Autodesk Inventor part; units mm, degrees
ref_plane "YZ Plane" through (0, 0, 0) normal (1, 0, 0) x (0, 1, 0)
ref_plane "XZ Plane" through (0, 0, 0) normal (0, 1, 0) x (-1, 0, 0)
ref_plane "XY Plane" through (0, 0, 0) normal (0, 0, 1) x (1, 0, 0)
sketch "Esboço1" plane through (0, 0, 0) normal (0, 1, 0) x (-1, 0, 0)
  line L0 (2.5876, 3.6816) -> (2.5876, -3.6816)
  line L1 (-2.5876, 3.6816) -> (-2.5876, -3.6816)
  arc A0 (2.5876, 3.6816) -> (-2.5876, 3.6816) centre (0, 0) ccw
  arc A1 (-2.5876, -3.6816) -> (2.5876, -3.6816) centre (0, 0) ccw
extrude "Extrusão1" add sketch "Esboço1" along normal blind 0.3
sketch "Esboço2" plane through (0, 0.3, 0) normal (0, 1, 0) x (1, 0, 0)
  circle A0 centre (0, 0) radius 3.5
  dimension "d3" = 7
extrude "Extrusão2" add sketch "Esboço2" along normal blind 5
properties part number "button"
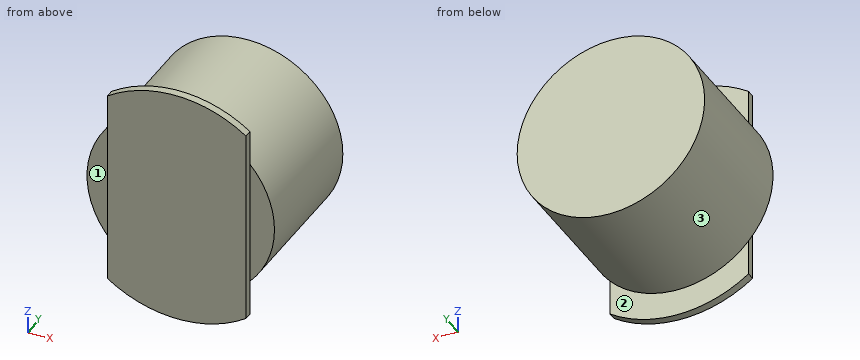
Design review of the part built by this model. Coordinates are the model's own, in mm. Face numbers are marked on the shaded views. A direction names the side the tool comes from. Round coordinates to 2 decimals unless told otherwise and drop trailing zeros. Write each loop counter-clockwise with the first axis right and the second up, starting at its lowest first coordinate (ties: lowest second). Pieces come first, ordered by that corner, then holes. Notation, with made-up numbers: (-6, 24.25) -> (50, 24.25) arc R24 ccw to (50, 38.25) -> close; hole circle Ø9 at (73, 50). An arc over 180 degrees is marked (long way). One line per item, written item: value. Start each with the question number.
Q1. Tool access review of the marked faces 1, 2 and 3: name each direction out of +Z, -Z, +X, -X, +Y, -Y from which nothing blocks a thin tool from reaching the whole face with its end or side.
Q2. To check wall thickness, follow probe 1 along Y at (x, z) = (-2, 4); probe 2 along X at (y, z) = (0.25, -2); probe 3 along Z at (x, y) = (0, 3.95). State the ranges of each line that lie inside material, in increasing order.
Q3. Add section B-B (y = 3). Give the boundary of the cut face in (x, z), then the cut area to 3 significant figures.
Q4. Add section A-A (x = 0). Give the boundary of the cut face in (y, z), then the cut area to 3 significant figures.
Q5. Add section C-C (x = 0.75). Give the boundary of the cut face in (y, z), then the cut area to 3 significant figures.
Q6. Insertion check: P1, Ø0.6, axis at x = 1, z = -3.5, coming from the +Y side; P2, Ø2, axis at x = 1.5, y = 0.5, coming from the +Z side; P3, Ø1, axis at x = -3.5, z = -1, coming from the -Y side; P4, Ø1.5, axis at y = 1, z = -1.5, coming from the -X side. Each pin has a flat end and moves straight along its axis. Give the tip position at first contact, or say it passes through.
Response:
1. face 1: +Z, -Z, -X, -Y
1. face 2: -Z, +Y
1. face 3: +Y
2. probe 1: y = 0 to 0.3
2. probe 2: x = -2.59 to 2.59
2. probe 3: z = -3.5 to 3.5
3. outline: circle Ø7 at (0, 0)
3. area: 38.5 mm^2
4. outline: (0, -4.5) -> (0.3, -4.5) -> (0.3, -3.5) -> (5.3, -3.5) -> (5.3, 3.5) -> (0.3, 3.5) -> (0.3, 4.5) -> (0, 4.5) -> close
4. area: 37.7 mm^2
5. outline: (0, -4.44) -> (0.3, -4.44) -> (0.3, -3.42) -> (5.3, -3.42) -> (5.3, 3.42) -> (0.3, 3.42) -> (0.3, 4.44) -> (0, 4.44) -> close
5. area: 36.8 mm^2
6. P1: stops at y = 5.3
6. P2: stops at z = 4.47
6. P3: stops at y = 0.3
6. P4: stops at x = -3.42
